Autodesk Inventor part; units mm, degrees
ref_plane "YZ Plane" through (0, 0, 0) normal (1, 0, 0) x (0, 1, 0)
ref_plane "XZ Plane" through (0, 0, 0) normal (0, 1, 0) x (-1, 0, 0)
ref_plane "XY Plane" through (0, 0, 0) normal (0, 0, 1) x (1, 0, 0)
sketch "Sketch1" plane through (0, 0, 0) normal (0, 0, 1) x (1, 0, 0)
  line L0 (0, 2) -> (3.2, 2)
  line L1 (3.2, 2) -> (3.2, 0)
  line L2 (3.2, 0) -> (12.5, 0)
  line L3 (12.5, 0) -> (12.5, 5)
  line L4 (12.5, 5) -> (0, 5)
  line L5 (0, 0) -> (0, 5) construction
  line L6 (0, 2) -> (-3.2, 2)
  line L7 (-3.2, 2) -> (-3.2, 0)
  line L8 (-3.2, 0) -> (-12.5, 0)
  line L9 (-12.5, 0) -> (-12.5, 5)
  line L10 (-12.5, 5) -> (0, 5)
  dimension "d0" = 3.2
  dimension "d1" = 2
  dimension "d2" = 9.3
  dimension "d3" = 5
extrude "Extrusion1" add sketch "Sketch1" along normal blind 43
sketch "Sketch2" plane through (-12.5, 5, 0) normal (0, 1, 0) x (1, 0, 0)
  circle A0 centre (12.5, -33) radius 1.25
  circle A1 centre (12.5, -10) radius 1.25
  line L0 (25, 0) -> (0, 0)
  line L1 (25, -43) -> (0, -43)
  point P0 (12.5, 0)
  dimension "d6" = 2.5
  dimension "d7" = 2.5
  dimension "d8" = 10
  dimension "d9" = 10
extrude "Extrusion2" cut sketch "Sketch2" against normal up to surface (3 mm away)
sketch "Sketch3" plane through (-12.5, 5, 0) normal (0, 1, 0) x (1, 0, 0)
  circle A0 centre (12.5, -33) radius 1.25
  circle A1 centre (12.5, -33) radius 3.5
  circle A2 centre (12.5, -10) radius 1.25
  circle A3 centre (12.5, -10) radius 3.5
  point P0 (12.5, 0)
  dimension "d12" = 7
  dimension "d13" = 7
extrude "Extrusion3" cut sketch "Sketch3" against normal blind 2
fillet "Fillet1" radius 5 6 edges at (-12.5, 2.5, 0) (12.5, 2.5, 0) (12.5, 2.5, 43) (-12.5, 2.5, 43) (12.5, 0, 21.5) (-12.5, 0, 21.5)
properties part number "Gripper 5-4"
The model under review builds one solid part; all positions refer to its coordinate system, in mm. A direction names the side the tool comes from. Give positions to 0.01 mm unless a question says otherwise; leave off trailing zeros. Write each loop counter-clockwise with the first axis right and the second up, starting at its lowest first coordinate (ties: lowest second). Pieces come first, ordered by that corner, then holes.
(1) Tool access review of faces 1 (the cylindrical face through (-10.32, 3.09, 0.87)), 2 (the flat face through (-3.2, 1, 21)), 3 (the cylindrical face through (-0.759, 4.014, 13.417)): name each direction out of +Z, -Z, +X, -X, +Y, -Y from which nothing blocks a thin tool from reaching the whole face with its end or side.
(2) The part is to be moulded in two halves that separate along Z. For faces 4 (the flat face through (0, 2, 21)), 5 (the cylindrical face through (-10.413, 3.091, 42.064)), 6 (the cylindrical face through (-0.46, 4.01, 29.53)), say which applies: released by +Z, released by -Z, zero draft, split by the parting line, or undercut.
(3) Consider section C-C, the plane y = 1.1. Give the boundary of the cut face in (x, z), and give its area (3 significant figures).
(4) To check wall thickness, follow L1, parallel to Z at x = 0, y = 4.1; L2, parallel to Y at x = 7.75, z = 24.5; L3, parallel to X at y = 1.8, z = 20. State the ranges of each line that lie inside material, in increasing order.
(5) Consider section A-A, the plane x = 0. Give the boundary of the cut face in (y, z), and give its area (3 significant figures).
(6) For P1, Ø1, axis at y = 1, z = 31.5, coming from the -X side; P2, Ø0.6, axis at y = 0.5, z = 23, coming from the -X side; P3, Ø3, axis at x = 0, z = 10, coming from the -Y side; P4, Ø1.5, axis at x = 1, y = 0.5, coming from the -Z side, all flat-tipped, find the tip position at first contact; note any pin that passes through.
Returned:
1. face 1: -Z, -X, +Y, -Y
1. face 2: +Z, -Z, -Y
1. face 3: +Y
2. face 4: zero draft
2. face 5: released by +Z
2. face 6: undercut
3. outline: (-10.63, 1.1) arc R5 ccw to (-7.5, 0) - (-3.2, 0) - (-3.2, 43) - (-7.5, 43) arc R5 ccw to (-10.63, 41.9) - close; (3.2, 0) - (7.5, 0) arc R5 ccw to (10.63, 1.1) - (10.63, 41.9) arc R5 ccw to (7.5, 43) - (3.2, 43) - close
3. area: 635 mm2
4. L1: z = 0 to 6.5, 13.5 to 29.5, 36.5 to 43
4. L2: y = 0.01 to 5
4. L3: x = -11.34 to -3.2, 3.2 to 11.34
5. outline: (2, 0) - (5, 0) - (5, 6.5) - (3, 6.5) - (3, 8.75) - (2, 8.75) - close; (2, 11.25) - (3, 11.25) - (3, 13.5) - (5, 13.5) - (5, 29.5) - (3, 29.5) - (3, 31.75) - (2, 31.75) - close; (2, 34.25) - (3, 34.25) - (3, 36.5) - (5, 36.5) - (5, 43) - (2, 43) - close
5. area: 96.0 mm2
6. P1: stops at x = -11.07
6. P2: stops at x = -10.21
6. P3: stops at y = 2
6. P4: passes through
